```python
from build123d import *

# Parameters (mm, degrees)
BOSS_EXTRUDE1_DEPTH = 2.015360823
CUT_EXTRUDE4_DEPTH  = 1
SKETCH14_W          = 0.787440713
SKETCH14_H          = 8.825897992
SKETCH14_H_2        = 7.775977042
SKETCH14_W_2        = 0.721820654
SKETCH14_H_3        = 6.168285585
SKETCH14_H_4        = 7.907217161
CUT_EXTRUDE8_DEPTH  = 2
SKETCH16_R          = 0.858720655
CUT_EXTRUDE9_DEPTH  = 2
SKETCH17_W          = 1.980286876
SKETCH17_H          = 0.530178386
SKETCH17_W_2        = 0.459340416
SKETCH17_H_2        = 3.773153417
SKETCH17_W_3        = 1.417450885
SKETCH17_H_3        = 0.52338797
SKETCH17_H_4        = 0.521784595
SKETCH17_W_4        = 3.263347093
BOSS_EXTRUDE5_DEPTH = 1
SKETCH18_R          = 0.400497452
BOSS_EXTRUDE6_DEPTH = 1


with BuildPart() as part:
    # Sketch1 → Boss-Extrude1 (new body)
    with BuildSketch(Plane(origin=(0, 0, 0), x_dir=(1, 0, 0), z_dir=(0, 1, 0))):
        Polygon((-24.716746523, 29.689845928), (-24.716746523, 27.490492708), (-24.716746523, 6.596637121), (-22.39957081, 4.279461407), (-5.708050839, 4.279461407), (-3.390875125, 6.596637121), (-3.390875125, 29.689845928), align=None)
    extrude(amount=BOSS_EXTRUDE1_DEPTH)

    # Sketch13 → Cut-Extrude4 (cut)
    with BuildSketch(Plane(origin=(0, 2.015360823, 0), x_dir=(1, 0, 0), z_dir=(0, 1, 0))):
        Polygon((-23.962439797, 28.911099467), (-23.962439797, 6.633089294), (-22.321938311, 4.992587808), (-5.851303397, 4.992587808), (-4.210801911, 6.633089294), (-4.210801911, 28.911099467), align=None)
    extrude(amount=-CUT_EXTRUDE4_DEPTH, mode=Mode.SUBTRACT)

    # Sketch14 → Cut-Extrude8 (cut)
    with BuildSketch(Plane(origin=(0, 1.015360823, 0), x_dir=(1, 0, 0), z_dir=(0, 1, 0))):
        with Locations((-22.978138906, 20.429706787)):
            Rectangle(SKETCH14_W, SKETCH14_H)
        with Locations((-22.978138906, 11.341328557)):
            Rectangle(SKETCH14_W, SKETCH14_H_2)
        with Locations((-5.621633189, 19.461810911)):
            Rectangle(SKETCH14_W_2, SKETCH14_H_3)
        with Locations((-5.621633189, 11.177278409)):
            Rectangle(SKETCH14_W_2, SKETCH14_H_4)
    extrude(amount=-CUT_EXTRUDE8_DEPTH, mode=Mode.SUBTRACT)

    # Sketch16 → Cut-Extrude9 (cut)
    with BuildSketch(Plane(origin=(0, 1.015360823, 0), x_dir=(1, 0, 0), z_dir=(0, 1, 0))):
        with Locations((-14.086620854, 6.698709353)):
            Circle(SKETCH16_R)
    extrude(amount=-CUT_EXTRUDE9_DEPTH, mode=Mode.SUBTRACT)

    # Sketch17 → Boss-Extrude5 (add)
    with BuildSketch(Plane(origin=(0, 1.015360823, 0), x_dir=(1, 0, 0), z_dir=(0, 1, 0))):
        Polygon((-6.60593408, 28.025228665), (-21.600117658, 28.025228665), (-21.600117658, 18.575940108), (-20.943917063, 18.575940108), (-20.943917063, 20.028920156), (-20.943917063, 20.559098542), (-20.943917063, 27.43464813), (-14.742821448, 27.43464813), (-14.283481032, 27.43464813), (-7.163704585, 27.43464813), (-7.163704585, 21.856943079), (-6.60593408, 21.856943079), align=None)
        with Locations((-19.953773625, 20.294009349)):
            Rectangle(SKETCH17_W, SKETCH17_H)
        with Locations((-14.51315124, 25.548071422)):
            Rectangle(SKETCH17_W_2, SKETCH17_H_2)
        Polygon((-20.943917063, 17.526019157), (-21.600117658, 17.526019157), (-21.600117658, 8.864171314), (-14.742821448, 8.864171314), (-14.742821448, 9.421941819), (-20.943917063, 9.421941819), align=None)
        Polygon((-7.163704585, 9.421941819), (-14.053810824, 9.421941819), (-14.053810824, 8.864171314), (-6.60593408, 8.864171314), (-6.60593408, 20.971072277), (-7.163704585, 20.971072277), (-7.163704585, 18.575940108), (-7.163704585, 18.054155513), (-7.163704585, 15.196507048), (-7.163704585, 14.673119078), align=None)
        with Locations((-7.872430028, 14.934813063)):
            Rectangle(SKETCH17_W_3, SKETCH17_H_3)
        with Locations((-7.872430028, 18.315047811)):
            Rectangle(SKETCH17_W_3, SKETCH17_H_4)
        Polygon((-14.283481032, 22.542256975), (-14.742821448, 22.542256975), (-14.742821448, 20.559098542), (-14.742821448, 20.028920156), (-14.742821448, 18.054155513), (-14.283481032, 18.054155513), (-9.478775763, 18.054155513), (-9.478775763, 18.575940108), (-14.283481032, 18.575940108), align=None)
        with Locations((-16.374494995, 20.294009349)):
            Rectangle(SKETCH17_W_4, SKETCH17_H)
        Polygon((-14.283481032, 18.054155513), (-14.742821448, 18.054155513), (-14.742821448, 14.673119078), (-9.478775763, 14.673119078), (-9.478775763, 15.181770577), (-14.283481032, 15.181770577), align=None)
    extrude(amount=BOSS_EXTRUDE5_DEPTH)

    # Sketch18 → Boss-Extrude6 (add)
    with BuildSketch(Plane(origin=(0, 1.015360823, 0), x_dir=(1, 0, 0), z_dir=(0, 1, 0))):
        with Locations((-23.010948935, 27.795558457)):
            Circle(SKETCH18_R)
        with Locations((-20.622593862, 6.426229891)):
            Circle(SKETCH18_R)
        with Locations((-5.293532892, 27.795558457)):
            Circle(SKETCH18_R)
        with Locations((-7.78709515, 6.426229891)):
            Circle(SKETCH18_R)
    extrude(amount=BOSS_EXTRUDE6_DEPTH)


solid = part.part
```
Verification items for the finished model (mm, model axes). A direction names the side the tool comes from. Round coordinates to 2 decimals unless told otherwise and drop trailing zeros. Write each loop counter-clockwise with the first axis right and the second up, starting at its lowest first coordinate (ties: lowest second). Pieces come first, ordered by that corner, then holes. Notation, with made-up numbers: (-3, 21.5) -> (56, 21.5) arc R15 ccw to (56, 30.5) -> close; hole circle Ø8 at (57.25, 39). An arc over 180 degrees is marked (long way). Write each question's results on one line, items separated by ' | '.
Q1. Thickness scan on probe 1 along Z at (x, y) = (-9, 1.75); probe 2 along X at (y, z) = (1.45, -18); probe 3 along X at (y, z) = (1.7, -23.5). Record the ranges inside material, lowest first.
Derived:
probe 1: z = -29.69 to -28.91, -28.03 to -27.43, -9.42 to -8.86, -4.99 to -4.28 | probe 2: x = -24.72 to -23.96, -14.74 to -14.28, -7.16 to -6.61, -4.21 to -3.39 | probe 3: x = -24.72 to -23.96, -21.6 to -20.94, -7.16 to -6.61, -4.21 to -3.39
Q2. Go/stop test with flat-tipped pins: pin 1 Ø1.5 at (x, z) = (-9, -25) entering from +Y; pin 2 Ø0.6 at (x, y) = (-23, 0.5) entering from +Z; pin 3 Ø1.5 at (x, z) = (-14.09, -6.7) entering from +Y. Record where each tip stops, or that it passes through.
Derived:
pin 1: stops at y = 1.02 | pin 2: stops at z = -4.58 | pin 3: passes through
Q3. Access from +Z, -Z, +X, -X, +Y, -Y to the whole of each face (thin tool, end or side, straight path). Record for faces 4 (the face through (-23, 2.015, -28)), 5 (the face through (-23.41, 1.51, -27.81)), 6 (the face through (-23.372, 0.5, -11.3)).
Derived:
face 4: +Z, -Z, +X, -X, +Y | face 5: +Y | face 6: +Y, -Y
Q4. Sectioned sample at C-C, the plane y = 0.3. Record the boundary of the cut face in (x, z).
Derived:
outline: (-24.72, -29.69) -> (-3.39, -29.69) -> (-3.39, -6.6) -> (-5.71, -4.28) -> (-22.4, -4.28) -> (-24.72, -6.6) -> close; hole (-23.37, -24.84) -> (-22.58, -24.84) -> (-22.58, -16.02) -> (-23.37, -16.02) -> close; hole (-23.37, -15.23) -> (-22.58, -15.23) -> (-22.58, -7.45) -> (-23.37, -7.45) -> close; hole circle Ø1.72 at (-14.09, -6.7); hole (-5.98, -22.55) -> (-5.26, -22.55) -> (-5.26, -16.38) -> (-5.98, -16.38) -> close; hole (-5.98, -15.13) -> (-5.26, -15.13) -> (-5.26, -7.22) -> (-5.98, -7.22) -> close
Q5. Sectioned sample at D-D, the plane x = -10. Record the boundary of the cut face in (y, z), and give its area (3 significant figures).
Derived:
outline: (0, -29.69) -> (2.02, -29.69) -> (2.02, -28.91) -> (1.02, -28.91) -> (1.02, -28.03) -> (2.02, -28.03) -> (2.02, -27.43) -> (1.02, -27.43) -> (1.02, -18.58) -> (2.02, -18.58) -> (2.02, -18.05) -> (1.02, -18.05) -> (1.02, -15.18) -> (2.02, -15.18) -> (2.02, -14.67) -> (1.02, -14.67) -> (1.02, -9.42) -> (2.02, -9.42) -> (2.02, -8.86) -> (1.02, -8.86) -> (1.02, -4.99) -> (2.02, -4.99) -> (2.02, -4.28) -> (0, -4.28) -> close | area: 29.5 mm²
Q6. Sectioned sample at B-B, the plane z = -26.5. Record the boundary of the cut face in (x, y), and give its area (3 significant figures).
Derived:
outline: (-24.72, 0) -> (-3.39, 0) -> (-3.39, 2.02) -> (-4.21, 2.02) -> (-4.21, 1.02) -> (-6.61, 1.02) -> (-6.61, 2.02) -> (-7.16, 2.02) -> (-7.16, 1.02) -> (-14.28, 1.02) -> (-14.28, 2.02) -> (-14.74, 2.02) -> (-14.74, 1.02) -> (-20.94, 1.02) -> (-20.94, 2.02) -> (-21.6, 2.02) -> (-21.6, 1.02) -> (-23.96, 1.02) -> (-23.96, 2.02) -> (-24.72, 2.02) -> close | area: 24.9 mm²
Q7. Sectioned sample at A-A, the plane x = -16.5. Record the boundary of the cut face in (y, z), and give its area (3 significant figures).
Derived:
outline: (0, -29.69) -> (2.02, -29.69) -> (2.02, -28.91) -> (1.02, -28.91) -> (1.02, -28.03) -> (2.02, -28.03) -> (2.02, -27.43) -> (1.02, -27.43) -> (1.02, -20.56) -> (2.02, -20.56) -> (2.02, -20.03) -> (1.02, -20.03) -> (1.02, -9.42) -> (2.02, -9.42) -> (2.02, -8.86) -> (1.02, -8.86) -> (1.02, -4.99) -> (2.02, -4.99) -> (2.02, -4.28) -> (0, -4.28) -> close | area: 29.0 mm²
Q8. Draft check along Z on faces 1 (the face through (-21.2, 2.015, -11.6)), 2 (the face through (-21.6, 1.5, -13.3)), 3 (the face through (-4.57, 0.99, -5.42)). Enter one of: released by +Z, released by -Z, zero draft, split by the parting line, or undercut.
Derived:
face 1: zero draft | face 2: undercut | face 3: released by +Z
